from build123d import *

# Parameters (mm, degrees)
F0_W      = 25.4
F0_H      = 7.62
F0_H_2    = 17.78
F1_DEPTH  = 5.08
F2_W      = 25.4
F2_H      = 3.81
F3_DEPTH  = 25.4
F4_W      = 25.4
F4_H      = 25.4
F5_DEPTH  = 5.08
F6_W      = 25.4
F6_H      = 15.24
F7_DEPTH  = 5.08
F9_DEPTH  = 2.54
F11_DEPTH = 2.54


with BuildPart() as f1:
    # F0 (on Top) → F1 (new body)
    with BuildSketch(Plane.XY):
        with Locations((-12.7, 3.81)):
            Rectangle(F0_W, F0_H)
        with Locations((-12.7, -8.89)):
            Rectangle(F0_W, F0_H_2)
    extrude(amount=F1_DEPTH)

    # F2 (on face) → F3 (join)
    with BuildSketch(Plane.XY.offset(5.08)):
        with Locations((-12.7, -15.875)):
            Rectangle(F2_W, F2_H)
        with Locations((-12.7, 5.715)):
            Rectangle(F2_W, F2_H)
    extrude(amount=F3_DEPTH)

    # F4 (on face) → F5 (join)
    with BuildSketch(Plane.XY.offset(30.48)):
        with Locations((-12.7, -5.08)):
            Rectangle(F4_W, F4_H)
    extrude(amount=F5_DEPTH)

    # F6 (on face) → F7 (join)
    with BuildSketch(Plane.XZ.offset(17.78)):
        with Locations((-12.7, 17.78)):
            Rectangle(F6_W, F6_H)
    extrude(amount=F7_DEPTH)

    # F8 (on face) → F9 (join)
    with BuildSketch(Plane.YZ):
        with BuildLine():
            Line((-20.32, 17.78), (-18.415, 17.78))
            Line((-18.415, 17.78), (-16.51, 17.78))
            ThreePointArc((-16.51, 17.78), (-18.415, 19.685), (-20.32, 17.78))
        make_face()
        with BuildLine():
            Line((-16.51, 17.78), (-18.415, 17.78))
            Line((-18.415, 17.78), (-20.32, 17.78))
            ThreePointArc((-20.32, 17.78), (-18.415, 15.875), (-16.51, 17.78))
        make_face()
    extrude(amount=F9_DEPTH)

    # F10 (on face) → F11 (join)
    with BuildSketch(Plane(origin=(-25.4, 0, 0), x_dir=(0, -1, 0), z_dir=(-1, 0, 0))):
        with BuildLine():
            ThreePointArc((16.51, 17.78), (18.415, 15.875), (20.32, 17.78))
            Line((20.32, 17.78), (18.415, 17.78))
            Line((18.415, 17.78), (16.51, 17.78))
        make_face()
        with BuildLine():
            Line((18.415, 17.78), (20.32, 17.78))
            ThreePointArc((20.32, 17.78), (18.415, 19.685), (16.51, 17.78))
            Line((16.51, 17.78), (18.415, 17.78))
        make_face()
    extrude(amount=F11_DEPTH)


solid = f1.part
Geometry check sheet. Reference: the model listing, model coordinates, mm. A direction names the side the tool comes from. Give positions to 0.01 mm unless a question says otherwise; leave off trailing zeros. Order: outer loops, then holes, each group sorted by start corner. A loop starts at its lowest first (then second) coordinate and runs counter-clockwise, first axis right, second up. Notation, with made-up numbers: (30, 36.5) - (50, 36.5) arc R14 cw to (50, 56.5) - close; hole circle Ø9 at (-40, 41.5). An arc over 180 degrees is marked (long way). Answer as a JSON object with one key per item and string values.
(1) Material ranges on line 1 (Z direction, x = -25, y = -12); line 2 (Y direction, x = -9.5, z = 12.5); line 3 (Y direction, x = -23, z = 10), recorded low to high.
Report:
{"line 1": "0 to 5.08, 30.48 to 35.56", "line 2": "-22.86 to -13.97, 3.81 to 7.62", "line 3": "-17.78 to -13.97, 3.81 to 7.62"}
(2) Cross-section at A-A (y = -10). Record the cut outline in (x, z), then the cut area to 3 significant figures.
Report:
{"outline": "(-25.4, 0) - (0, 0) - (0, 5.08) - (-25.4, 5.08) - close; (-25.4, 30.48) - (0, 30.48) - (0, 35.56) - (-25.4, 35.56) - close", "area": "258 mm^2"}
(3) Cross-section at D-D (z = 24.5). Record the cut outline in (x, y).
Report:
{"outline": "(-25.4, -22.86) - (0, -22.86) - (0, -13.97) - (-25.4, -13.97) - close; (-25.4, 3.81) - (0, 3.81) - (0, 7.62) - (-25.4, 7.62) - close"}
(4) Tool access check on faces 1 (the flat face through (-13, -5, 35.56)), 2 (the flat face through (-13, -5, 30.48)), 3 (the flat face through (-13, -20, 10.16)), 4 (the cylindrical face through (1.252, -17.011, 16.493)), 5 (the flat face through (-13, -20, 25.4)). Record the directions out of +Z, -Z, +X, -X, +Y, -Y that give a thin tool (end or side, any length) a straight path to the whole face; none if there is none.
Report:
{"face 1": "+Z, +X, -X, +Y, -Y", "face 2": "+X, -X", "face 3": "-Z, +X, -X, -Y", "face 4": "+X", "face 5": "+Z, +X, -X, -Y"}
(5) Cross-section at B-B (z = 17.78). Record the cut outline in (x, y), then the cut area to 3 significant figures.
Report:
{"outline": "(-27.94, -20.32) - (-25.4, -20.32) - (-25.4, -22.86) - (0, -22.86) - (0, -20.32) - (2.54, -20.32) - (2.54, -16.51) - (0, -16.51) - (0, -13.97) - (-25.4, -13.97) - (-25.4, -16.51) - (-27.94, -16.51) - close; (-25.4, 3.81) - (0, 3.81) - (0, 7.62) - (-25.4, 7.62) - close", "area": "342 mm^2"}
(6) Cross-section at C-C (x = -12.5). Record the cut outline in (y, z).
Report:
{"outline": "(-22.86, 10.16) - (-17.78, 10.16) - (-17.78, 0) - (7.62, 0) - (7.62, 35.56) - (-17.78, 35.56) - (-17.78, 25.4) - (-22.86, 25.4) - close; hole (-13.97, 5.08) - (3.81, 5.08) - (3.81, 30.48) - (-13.97, 30.48) - close"}
(7) Depth check by flat-ended pin: pin 1 Ø10 at (y, z) = (-9.5, 17.5) entering from -X; pin 2 Ø1.5 at (x, y) = (-17, -20) entering from -Z; pin 3 Ø8 at (x, z) = (-8.5, 30.5) entering from -Y. Enter the tip coordinate at first touch or a pass-through.
Report:
{"pin 1": "x = -25.4", "pin 2": "z = 10.16", "pin 3": "y = -17.78"}
(8) Draft check along Z on faces 6 (the cylindrical face through (-26.65, -16.51, 17.86)), 7 (the flat face through (-13, -13.97, 18)), 8 (the flat face through (-13, -17.78, 5)). Enter one of: released by +Z, released by -Z, zero draft, split by the parting line, or undercut.
Report:
{"face 6": "split by the parting line", "face 7": "undercut", "face 8": "zero draft"}
